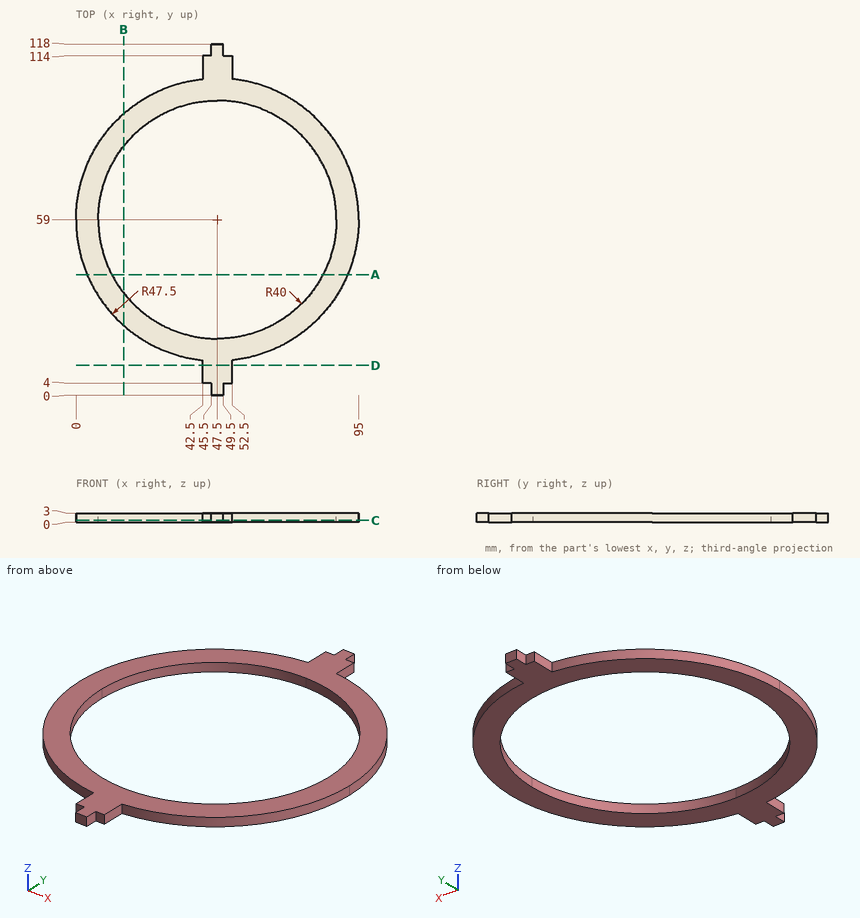
Geometry check sheet. Reference: drawing and pictorial views, mm from the part's lowest x, y, z. Round coordinates to 2 decimals unless told otherwise and drop trailing zeros. Loops run counter-clockwise (first coordinate to the right, second up) from the corner with the lowest first, then second, coordinate; pieces in that order, holes last. Notation, with made-up numbers: (-8.75, 47) - (18.25, 47) arc R12 ccw to (18.25, 56) - close; hole circle Ø8 at (52.25, 65). An arc over 180 degrees is marked (long way). Answer in a Markdown table with one row per item. Add a question column.
Q1. Material ranges on line 1 (X direction, y = 112, z = 1.45); line 2 (Y direction, x = 44.5, z = 1); line 3 (X direction, y = 25, z = 1.5), recorded low to high.
Q2. Section check A-A on y = 40.5. Enter the section's corners in (x, z).
Q3. Gauge pin test, flat ends, axial feed: pin 1 (1.5 mm diameter, centred on y = 65, z = 1, fed in from -X); pin 2 (1 mm diameter, centred on y = 76.5, z = 0.5, fed in from -X); pin 3 (1.5 mm diameter, centred on x = 51, z = 2, fed in from -Y). Record the tip position at first contact, or that the pin passes through.
Q4. Section check D-D on y = 10. Enter the section's corners in (x, z), plus the area to 3 significant figures.
Q5. Section check B-B on x = 16. Enter the section's corners in (y, z), plus the area to 3 significant figures.
Q6. Section check C-C on z = 0.6. Enter the section's corners in (x, y).
Found:
| question | item | result |
|---|---|---|
| 1 | line 1 | x = 42.5 to 52.5 |
| 1 | line 2 | y = 4 to 19.11, 98.89 to 114 |
| 1 | line 3 | x = 14.33 to 26.43, 68.57 to 80.67 |
| 2 | outline | (3.75, 0) - (12.04, 0) - (12.04, 3) - (3.75, 3) - close; (82.96, 0) - (91.25, 0) - (91.25, 3) - (82.96, 3) - close |
| 3 | pin 1 | stops at x = 0.29 |
| 3 | pin 2 | stops at x = 3.15 |
| 3 | pin 3 | stops at y = 4 |
| 4 | outline | (42.5, 0) - (52.5, 0) - (52.5, 3) - (42.5, 3) - close |
| 4 | area | 30.0 mm² |
| 5 | outline | (23.45, 0) - (34.35, 0) - (34.35, 3) - (23.45, 3) - close; (83.65, 0) - (94.55, 0) - (94.55, 3) - (83.65, 3) - close |
| 5 | area | 65.4 mm² |
| 6 | outline | (42.5, 4) - (45.5, 4) - (45.5, 0) - (49.5, 0) - (49.5, 4) - (52.5, 4) - (52.5, 11.76) arc R47.5 ccw to (52.5, 106.24) - (52.5, 114) - (49.5, 114) - (49.5, 118) - (45.5, 118) - (45.5, 114) - (42.5, 114) - (42.5, 106.24) arc R47.5 ccw to (42.5, 11.76) - close; hole (7.5, 59) arc R40 ccw to (47.5, 19) arc R40 ccw to (87.5, 59) arc R40 ccw to (47.5, 99) arc R40 ccw to start |
